Geometry: see drawing. Coordinates: mm, zero at the bounding-box minimum. A direction names the side the tool comes from. Coordinates: 2 decimals unless noted, no trailing zeros. Order: outer loops, then holes, each group sorted by start corner. A loop starts at its lowest first (then second) coordinate and runs counter-clockwise, first axis right, second up. Notation, with made-up numbers: (-9.75, 58) -> (1.25, 58) arc R20 ccw to (1.25, 88) -> close; hole circle Ø11 at (70, -29.75). An arc over 180 degrees is marked (long way). Use one line per item in the form item = value.
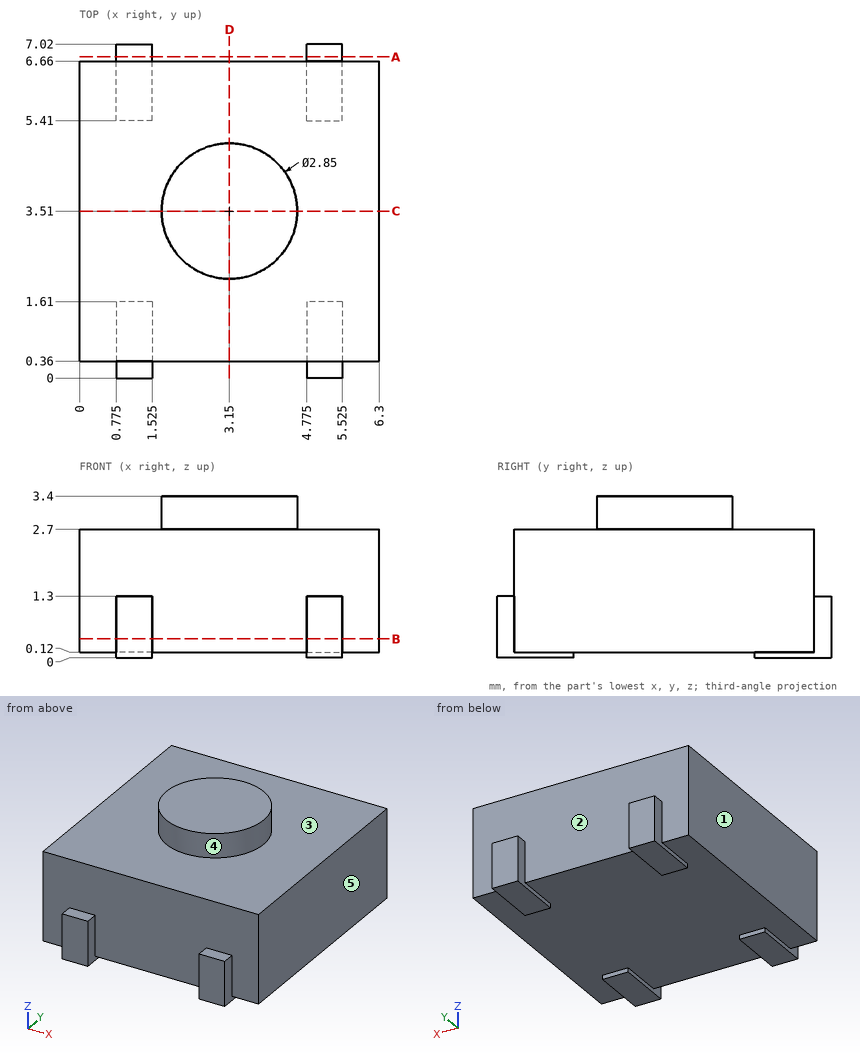
1) Section A-A, the plane y = 6.75. Output: boundary loops of the cut face in (x, z) (3 decimals), and give its area (3 significant figures).
Results found:
outline = (0.775, 0) -> (1.525, 0) -> (1.525, 1.3) -> (0.775, 1.3) -> close; (4.775, 0) -> (5.525, 0) -> (5.525, 1.3) -> (4.775, 1.3) -> close
area = 1.95 mm2
2) Access query for the marked faces 4 and 5. Directions: +Z, -Z, +X, -X, +Y, -Y. A direction counts if a zero-diameter tool reaches every point of the face in a straight line with its end or side. Return the directions, or none.
Results found:
face_4 = +Z
face_5 = +Z, -Z, +X, +Y, -Y
3) Section C-C, the plane y = 3.51. Output: boundary loops of the cut face in (x, z) (3 decimals), and give its area (3 significant figures).
Results found:
outline = (0, 0.12) -> (6.3, 0.12) -> (6.3, 2.7) -> (4.575, 2.7) -> (4.575, 3.4) -> (1.725, 3.4) -> (1.725, 2.7) -> (0, 2.7) -> close
area = 18.2 mm2
4) Pull-direction query (X, two-part tool) for the marked faces 1, 2 and 3; classes: released by +X, released by -X, zero draft, split by the parting line, or undercut.
Results found:
face_1 = released by -X
face_2 = undercut
face_3 = zero draft
5) Section B-B, the plane z = 0.4. Output: boundary loops of the cut face in (x, y) (3 decimals).
Results found:
outline = (0, 0.36) -> (0.775, 0.36) -> (0.775, 0) -> (1.525, 0) -> (1.525, 0.36) -> (4.775, 0.36) -> (4.775, 0) -> (5.525, 0) -> (5.525, 0.36) -> (6.3, 0.36) -> (6.3, 6.66) -> (5.525, 6.66) -> (5.525, 7.02) -> (4.775, 7.02) -> (4.775, 6.66) -> (1.525, 6.66) -> (1.525, 7.02) -> (0.775, 7.02) -> (0.775, 6.66) -> (0, 6.66) -> close
6) Section D-D, the plane x = 3.15. Output: boundary loops of the cut face in (y, z) (3 decimals).
Results found:
outline = (0.36, 0.12) -> (6.66, 0.12) -> (6.66, 2.7) -> (4.935, 2.7) -> (4.935, 3.4) -> (2.085, 3.4) -> (2.085, 2.7) -> (0.36, 2.7) -> close
7) Material intervals for probe 1 along Y at (x, z) = (3, 1.8); probe 2 along Z at (x, y) = (0.75, 4.5); probe 3 along Z at (x, y) = (3, 4), sorted ascending. Write a range as from..to.
Results found:
probe_1 = 0.36..6.66
probe_2 = 0.12..2.7
probe_3 = 0.12..3.4
